Job drawing, mm, ordinate dimensions from the low corner. One solid piece. Give positions to 0.01 mm unless a question says otherwise; leave off trailing zeros. Loops run counter-clockwise (first coordinate to the right, second up) from the corner with the lowest first, then second, coordinate; pieces in that order, holes last. Notation, with made-up numbers: (57.25, 8.5) - (71.25, 8.5) arc R29 cw to (71.25, 43.5) - close; hole circle Ø4 at (84, 78.25). An arc over 180 degrees is marked (long way). Answer as CSV lines item,"result". Start each with the question number.
Item 1: Saw through at B-B on x = 30. Give the cut face in (y, z) (1 decimal).
Item 2: Pull direction Y, two halves, no side cores. Call the marked faces 1, 2 and 3: pulls with the +Y half, pulls with the -Y half, needs draft (parallel to the pull), parting line crosses it, or undercut.
Item 3: Saw through at D-D on x = 40. Give the cut face in (y, z) (1 decimal).
Item 4: Saw through at C-C on z = 2.6. State how many separate pieces and enclosed holes the cut face has, plus the area to 3 significant figures.
Item 5: Pin check, flat tips, straight feed: pin 1 (1.9 mm diameter, centred on x = 35.65, y = 14.48, fed in from +Z); pin 2 (4 mm diameter, centred on x = 8.8, y = 29.98, fed in from -Z); pin 3 (1 mm diameter, centred on y = 38, z = 2, fed in from +X); pin 4 (1.5 mm diameter, centred on x = 32.5, z = 2, fed in from -Y) (1 decimal). Stop position of each tip, or through.
Item 6: Drill centre lines: L1, parallel to X at y = 29.5, z = 1.3 (1 decimal); L2, parallel to Y at x = 37, z = 1.3 (1 decimal); L3, parallel to Y at x = 10, z = 0.2 (1 decimal). Where is each one in solid material? Low to high. Write a range as from..to.
Item 7: Saw through at A-A on y = 26.5. Give the cut face in (x, z) (1 decimal).
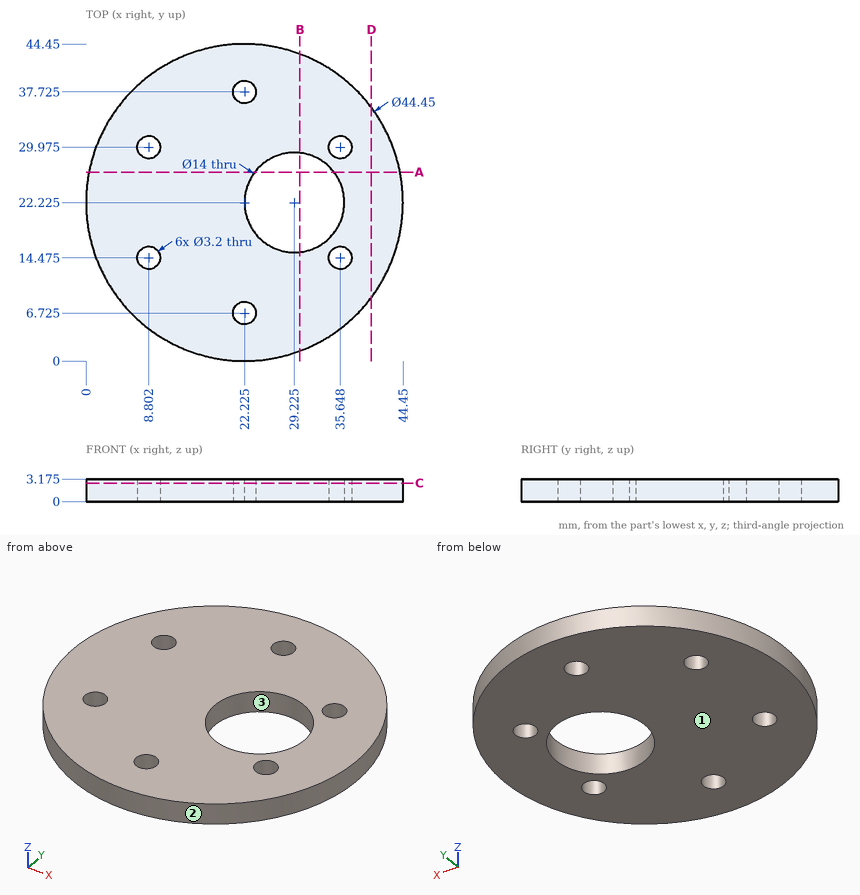
Responses:
1,outline,"(1.4, 0) - (15.3, 0) - (15.3, 3.2) - (1.4, 3.2) - close; (29.2, 0) - (43, 0) - (43, 3.2) - (29.2, 3.2) - close"
2,face 1,"needs draft"
2,face 2,"parting line crosses it"
2,face 3,"undercut"
3,outline,"(8.9, 0) - (35.6, 0) - (35.6, 3.2) - (8.9, 3.2) - close"
4,separate pieces,"1"
4,enclosed holes,"7"
4,area,"1,350 mm2"
5,pin 1,"through"
5,pin 2,"z = 0"
5,pin 3,"x = 38.37"
5,pin 4,"y = 2.1"
6,L1,"1.2..7.3, 10.3..34.1, 37.2..43.2"
6,L2,"5.6..13.6, 15.3..29.1, 30.8..38.8"
6,L3,"3.7..13.4, 15.5..28.9, 31..40.8"
7,outline,"(0.4, 0) - (23.7, 0) - (23.7, 3.2) - (0.4, 3.2) - close; (34.8, 0) - (44, 0) - (44, 3.2) - (34.8, 3.2) - close"
